The listing builds one solid part. Answer for the finished solid, in the listing's coordinates (mm). A direction names the side the tool comes from. Give positions to 0.01 mm unless a question says otherwise; leave off trailing zeros. Write each loop counter-clockwise with the first axis right and the second up, starting at its lowest first coordinate (ties: lowest second). Pieces come first, ordered by that corner, then holes. Notation, with made-up numbers: M 31,-6.75 L 51,-6.75 A25 cw 51,10.25 Z; hole C 76.5,21.25 d2. An arc over 180 degrees is marked long. Answer as a JSON object with one key per item and string values.
```python
from build123d import *

# Parameters (mm, degrees)
SKETCH_1_R          = 3.2
SKETCH_1_R_2        = 20
EXTRUDE_1_DEPTH     = 12
FILLET_1_R          = 10
CHAMFER_1_SIZE      = 3
SKETCH_2_R          = 5.5
CUT_EXTRUDE_1_DEPTH = 5


with BuildPart() as part:
    # 草图1 → 凸台-拉伸1 (new body)
    with BuildSketch(Plane.XY):
        Polygon((50, 40), (-50, 40), (-65, 40), (-65, -40), (-50, -40), (50, -40), (65, -40), (65, 40), align=None)
        with Locations((-50, -25)):
            Circle(SKETCH_1_R, mode=Mode.SUBTRACT)
        with Locations((-40, -20)):
            Circle(SKETCH_1_R, mode=Mode.SUBTRACT)
        with Locations((40, -20)):
            Circle(SKETCH_1_R, mode=Mode.SUBTRACT)
        with Locations((50, -25)):
            Circle(SKETCH_1_R, mode=Mode.SUBTRACT)
        with Locations((-50, 25)):
            Circle(SKETCH_1_R, mode=Mode.SUBTRACT)
        with Locations((-40, 20)):
            Circle(SKETCH_1_R, mode=Mode.SUBTRACT)
        Circle(SKETCH_1_R_2, mode=Mode.SUBTRACT)
        with Locations((40, 20)):
            Circle(SKETCH_1_R, mode=Mode.SUBTRACT)
        with Locations((50, 25)):
            Circle(SKETCH_1_R, mode=Mode.SUBTRACT)
    extrude(amount=EXTRUDE_1_DEPTH)

    # 圆角1
    fillet_1_edges = [part.edges().sort_by_distance(p)[0] for p in [
        (-65, -40, 6),
        (-65, 40, 6),
        (65, 40, 6),
        (65, -40, 6),
    ]]
    fillet(fillet_1_edges, radius=FILLET_1_R)

    # 倒角1
    chamfer_1_edges = [part.edges().sort_by_distance(p)[0] for p in [
        (-20, 0, 0),
    ]]
    chamfer(chamfer_1_edges, length=CHAMFER_1_SIZE)

    # 草图2 → 切除-拉伸1 (cut)
    with BuildSketch(Plane.XY.offset(12)):
        with Locations((-40, 20)):
            Circle(SKETCH_2_R)
        with Locations((-40, -20)):
            Circle(SKETCH_2_R)
        with Locations((40, 20)):
            Circle(SKETCH_2_R)
        with Locations((40, -20)):
            Circle(SKETCH_2_R)
    extrude(amount=-CUT_EXTRUDE_1_DEPTH, mode=Mode.SUBTRACT)


solid = part.part
```
1. For faces 1 (the cylindrical face through (37.461, 18.053, 3.451)), 2 (the cylindrical face through (34.505, -19.758, 9.535)), determine the directions among +Z, -Z, +X, -X, +Y, -Y from which every point of the face is accessible in a straight line to the end or side of a thin tool.
Verdict:
{"face 1": "+Z, -Z", "face 2": "+Z"}
2. A cutting plane is placed at D-D, the plane x = 50. Give the vertices of the cut face in (y, z), plus the area to 3 significant figures.
Verdict:
{"outline": "M -40,0 L -28.2,0 L -28.2,12 L -40,12 Z; M -21.8,0 L 21.8,0 L 21.8,12 L -21.8,12 Z; M 28.2,0 L 40,0 L 40,12 L 28.2,12 Z", "area": "806 mm2"}
3. The mould has two halves that part along X. Classify faces 3 (the flat face through (-1, -40, 6)), 4 (the cylindrical face through (47.461, -26.947, 5.916)), 5 (the cylindrical face through (61.99, -37.15, 6.08)): released by +X, released by -X, zero draft, split by the parting line, or undercut.
Verdict:
{"face 3": "zero draft", "face 4": "undercut", "face 5": "released by +X"}
4. Flat-ended cylindrical pins translate along their axes: pin 1 (3.5 mm diameter, centred on x = -41, y = -22.5, fed in from +Z); pin 2 (9 mm diameter, centred on x = 40, y = -20, fed in from -Z). Find the tip coordinate at first contact, or state that the pin passes through.
Verdict:
{"pin 1": "stops at z = 7", "pin 2": "stops at z = 0"}
5. A cutting plane is placed at A-A, the plane x = 0. Give the vertices of the cut face in (y, z), plus the area to 3 significant figures.
Verdict:
{"outline": "M -40,0 L -23,0 L -20,3 L -20,12 L -40,12 Z; M 20,3 L 23,0 L 40,0 L 40,12 L 20,12 Z", "area": "471 mm2"}
6. Consider line 1 along Y through (x, z) = (-50, 7.75); line 2 along Y through (x, z) = (40, 9.5); line 3 along X through (y, z) = (-17.5, 5). Determine where each line is inside the solid, lowest interval first.
Verdict:
{"line 1": "y = -40 to -28.2, -21.8 to 21.8, 28.2 to 40", "line 2": "y = -40 to -25.5, -14.5 to 14.5, 25.5 to 40", "line 3": "x = -65 to -42, -38 to -9.68, 9.68 to 38, 42 to 65"}
7. A cutting plane is placed at B-B, the plane y = 0. Give the vertices of the cut face in (x, z).
Verdict:
{"outline": "M -65,0 L -23,0 L -20,3 L -20,12 L -65,12 Z; M 20,3 L 23,0 L 65,0 L 65,12 L 20,12 Z"}
8. A cutting plane is placed at C-C, the plane z = 8.75. Count the separate pieces of the cut face and the enclosed holes in it, plus the area to 3 significant figures.
Verdict:
{"separate pieces": "1", "enclosed holes": "9", "area": "8,550 mm2"}
